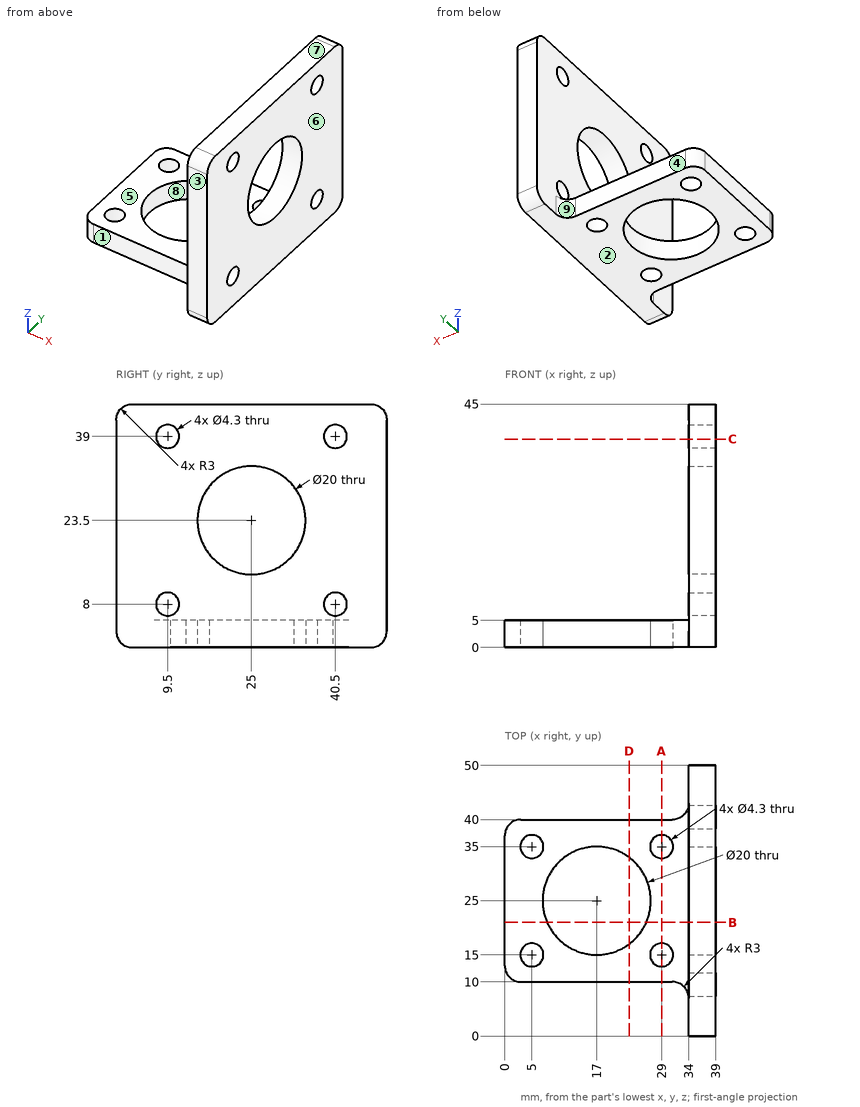
For this review, use the dimensioned drawing (mm, ordinates from the lowest corner) and the shaded views. A direction names the side the tool comes from. Round coordinates to 2 decimals unless told otherwise and drop trailing zeros. Write each loop counter-clockwise with the first axis right and the second up, starting at its lowest first coordinate (ties: lowest second). Pieces come first, ordered by that corner, then holes. Notation, with made-up numbers: (-3.5, 31) - (21.5, 31) arc R26 cw to (21.5, 62) - close; hole circle Ø7 at (3.25, 81.5). An arc over 180 degrees is marked (long way). Use a Markdown table: item, result.
Q1. We need section C-C (z = 38.5). Give the boundary of the cut face in (x, y).
Derived:
| item | result |
|---|---|
| outline | (34, 0) - (39, 0) - (39, 7.41) - (34, 7.41) - close; (34, 11.59) - (39, 11.59) - (39, 38.41) - (34, 38.41) - close; (34, 42.59) - (39, 42.59) - (39, 50) - (34, 50) - close |
Q2. The part is to be moulded in two halves that separate along X. For the marked faces 6, 7, 8 and 9, say which applies: pulls with the +X half, pulls with the -X half, needs draft (parallel to the pull), parting line crosses it, or undercut.
Derived:
| item | result |
|---|---|
| face 6 | pulls with the +X half |
| face 7 | needs draft |
| face 8 | undercut |
| face 9 | pulls with the -X half |
Q3. Wall thickness on line 1 along Y through (x, z) = (5, 3); line 2 along Y through (x, z) = (37.4, 8); line 3 along X through (y, z) = (3, 22): over which ranges is each line inside the solid? List them lowest first.
Derived:
| item | result |
|---|---|
| line 1 | y = 10 to 12.85, 17.15 to 32.85, 37.15 to 40 |
| line 2 | y = 0 to 7.35, 11.65 to 38.35, 42.65 to 50 |
| line 3 | x = 34 to 39 |
Q4. Clearance check with flat-ended pins moving along their axes: pin 1 (4 mm diameter, centred on x = 17, z = 3, fed in from +Y); pin 2 (5.5 mm diameter, centred on x = 29, y = 15, fed in from +Z); pin 3 (7 mm diameter, centred on y = 9.5, z = 39, fed in from -X). State where each tip first meets the part, or that it passes through.
Derived:
| item | result |
|---|---|
| pin 1 | stops at y = 40 |
| pin 2 | stops at z = 5 |
| pin 3 | stops at x = 34 |
Q5. Machinability: for the marked faces 1, 2, 3, 4 and 5, which of the approach directions +Z, -Z, +X, -X, +Y, -Y give a long, thin tool a straight path to every point of the face, cutting with its end or side? Answer none if there is none.
Derived:
| item | result |
|---|---|
| face 1 | +Z, -Z, -X, -Y |
| face 2 | -Z, +X, -X, +Y, -Y |
| face 3 | +Z, -Z, +X, -X, -Y |
| face 4 | +Z, -Z, -X, +Y |
| face 5 | +Z, -X, +Y, -Y |
Q6. We need section D-D (x = 23). Give the boundary of the cut face in (y, z).
Derived:
| item | result |
|---|---|
| outline | (10, 0) - (17, 0) - (17, 5) - (10, 5) - close; (33, 0) - (40, 0) - (40, 5) - (33, 5) - close |
Q7. We need section B-B (y = 21). Give the boundary of the cut face in (x, z).
Derived:
| item | result |
|---|---|
| outline | (0, 0) - (7.83, 0) - (7.83, 5) - (0, 5) - close; (26.17, 0) - (39, 0) - (39, 14.33) - (34, 14.33) - (34, 5) - (26.17, 5) - close; (34, 32.67) - (39, 32.67) - (39, 45) - (34, 45) - close |
Q8. We need section A-A (x = 29). Give the boundary of the cut face in (y, z), plus the area to 3 significant figures.
Derived:
| item | result |
|---|---|
| outline | (10, 0) - (12.85, 0) - (12.85, 5) - (10, 5) - close; (17.15, 0) - (32.85, 0) - (32.85, 5) - (17.15, 5) - close; (37.15, 0) - (40, 0) - (40, 5) - (37.15, 5) - close |
| area | 107 mm2 |
